Part model, mm, in its own coordinate system. A direction names the side the tool comes from. Coordinates: 2 decimals unless noted, no trailing zeros. Loops run counter-clockwise (first coordinate to the right, second up) from the corner with the lowest first, then second, coordinate; pieces in that order, holes last. Notation, with made-up numbers: M 53.5,-14 L 60.5,-14 A13 cw 60.5,5 Z; hole C 10.5,-19.75 d10. An arc over 180 degrees is marked long. Use a Markdown table: item, result. Add a question column.
1) Band-saw the part on B-B (y = -69.85). List the corners of the cut face in (x, z) (3 decimals).
2) Pull direction Y, two halves, no side cores. Call faces 4 (the flat face through (78, -38, 0)), 5 (the flat face through (152, -25.193, 5)), 6 (the cylindrical face through (5.9, -8.2, 0.8)): released by +Y, released by -Y, zero draft, split by the parting line, or undercut.
3) Band-saw the part on A-A (x = 152.4). List the corners of the cut face in (y, z) (3 decimals).
4) Tool access for faces 1 (the flat face through (43, -36, 4.877)), 2 (the flat face through (152, -45.767, 5)), 3 (the flat face through (43, -54.024, 3)): list every direction of +Z, -Z, +X, -X, +Y, -Y with a clear straight run to the whole face (end or side of a thin tool).
5) Band-saw the part on C-C (y = -52). List the corners of the cut face in (x, z), plus the area to 3 significant figures.
6) Wall check: probe 1 along Y at (x, z) = (152.4, 0.6) (3 decimals); probe 2 along X at (y, z) = (-69.85, 0.45) (3 decimals); probe 3 along X at (y, z) = (-40, 2.5). Give the ranges that are in metal, low to high. Write a range as from..to.
7) Pin check, flat tips, straight feed: pin 1 Ø1 at (y, z) = (-43, 4.5) entering from -X; pin 2 Ø3.5 at (x, y) = (152.4, -69.85) entering from -Z; pin 3 Ø1.5 at (x, y) = (83.5, -22) entering from +Z; pin 4 Ø2.5 at (x, z) = (155, 5.5) entering from +Y. Stop position of each tip, or through.
8) Band-saw the part on D-D (x = 35.5). List the corners of the cut face in (y, z), plus the area to 3 significant figures.
from build123d import *

# Parameters (mm, degrees)
SKETCH1_W          = 158.75
SKETCH1_H          = 76.2
EXTRUDE1_DEPTH     = 1.5748
SKETCH2_R          = 1.905
CUT_EXTRUDE2_DEPTH = 1.5748
SKETCH4_R          = 0.65
CUT_EXTRUDE3_DEPTH = 1.5748
SKETCH5_W          = 34.600619195
SKETCH5_H          = 36.173374613
EXTRUDE2_DEPTH     = 3.302
SKETCH6_W          = 13.081
SKETCH6_H          = 20.574
EXTRUDE3_DEPTH     = 7.874


with BuildPart() as part:
    # Sketch1 → Extrude1 (new body)
    with BuildSketch(Plane.XY):
        with Locations((79.375, -38.1)):
            Rectangle(SKETCH1_W, SKETCH1_H)
    extrude(amount=EXTRUDE1_DEPTH)

    # Sketch2 → Cut-Extrude2 (cut)
    with BuildSketch(Plane.XY.offset(1.5748)):
        with Locations((152.4, -6.35)):
            Circle(SKETCH2_R)
        with Locations((6.35, -6.35)):
            Circle(SKETCH2_R)
        with Locations((152.4, -69.85)):
            Circle(SKETCH2_R)
        with Locations((6.35, -69.85)):
            Circle(SKETCH2_R)
    extrude(amount=-CUT_EXTRUDE2_DEPTH, mode=Mode.SUBTRACT)

    # Sketch4 → Cut-Extrude3 (cut)
    with BuildSketch(Plane.XY.offset(1.5748)):
        with Locations((7.55, -19.234912)):
            Circle(SKETCH4_R)
        with Locations((7.55, -56.965088)):
            Circle(SKETCH4_R)
        with BuildLine():
            Line((0, -16.335006), (4.95, -16.335006))
            ThreePointArc((4.95, -16.335006), (5.657106781, -16.627899219), (5.95, -17.335006))
            Line((5.95, -17.335006), (5.95, -58.865006))
            ThreePointArc((5.95, -58.865006), (5.657106781, -59.572112781), (4.95, -59.865006))
            Line((4.95, -59.865006), (0, -59.865006))
            Line((0, -59.865006), (0, -16.335006))
        make_face()
    extrude(amount=-CUT_EXTRUDE3_DEPTH, mode=Mode.SUBTRACT)

    # Sketch5 → Extrude2 (add)
    with BuildSketch(Plane.XY.offset(1.5748)):
        with Locations((43.434262125, -35.937461301)):
            Rectangle(SKETCH5_W, SKETCH5_H)
    extrude(amount=EXTRUDE2_DEPTH)

    # Sketch6 → Extrude3 (add)
    with BuildSketch(Plane.XY.offset(1.5748)):
        with Locations((152.2095, -35.480182663)):
            Rectangle(SKETCH6_W, SKETCH6_H)
    extrude(amount=EXTRUDE3_DEPTH)


solid = part.part
Entries:
| question | item | result |
|---|---|---|
| 1 | outline | M 0,0 L 4.445,0 L 4.445,1.575 L 0,1.575 Z; M 8.255,0 L 150.495,0 L 150.495,1.575 L 8.255,1.575 Z; M 154.305,0 L 158.75,0 L 158.75,1.575 L 154.305,1.575 Z |
| 2 | face 4 | zero draft |
| 2 | face 5 | released by +Y |
| 2 | face 6 | undercut |
| 3 | outline | M -76.2,0 L -71.755,0 L -71.755,1.575 L -76.2,1.575 Z; M -67.945,0 L -8.255,0 L -8.255,1.575 L -25.193,1.575 L -25.193,9.449 L -45.767,9.449 L -45.767,1.575 L -67.945,1.575 Z; M -4.445,0 L 0,0 L 0,1.575 L -4.445,1.575 Z |
| 4 | face 1 | +Z, -X, +Y, -Y |
| 4 | face 2 | +Z, +X, -Y |
| 4 | face 3 | +Z, +X, -X, -Y |
| 5 | outline | M 5.95,0 L 158.75,0 L 158.75,1.57 L 60.73,1.57 L 60.73,4.88 L 26.13,4.88 L 26.13,1.57 L 5.95,1.57 Z |
| 5 | area | 355 mm2 |
| 6 | probe 1 | -76.2..-71.755, -67.945..-8.255, -4.445..0 |
| 6 | probe 2 | 0..4.445, 8.255..150.495, 154.305..158.75 |
| 6 | probe 3 | 26.13..60.73, 145.67..158.75 |
| 7 | pin 1 | x = 26.13 |
| 7 | pin 2 | through |
| 7 | pin 3 | z = 1.57 |
| 7 | pin 4 | y = -25.19 |
| 8 | outline | M -76.2,0 L 0,0 L 0,1.57 L -17.85,1.57 L -17.85,4.88 L -54.02,4.88 L -54.02,1.57 L -76.2,1.57 Z |
| 8 | area | 239 mm2 |
